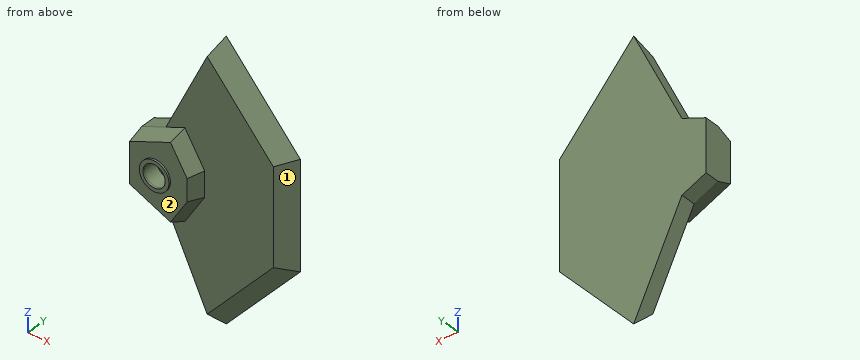
from build123d import *

# Parameters (mm, degrees)
F1_DEPTH      = 8
F1_TAPER      = -20
F2_W          = 14.830423519
F2_H          = 54.1627034545
F3_DEPTH      = 8.0010001
F4_R          = 6
F5_DEPTH      = 8.0010001
F5_DEPTH_BACK = 77
F4_R_2        = 8
F6_DEPTH      = 1
F9_DEPTH      = 8
F10_SIZE      = 7.99999


# Not quite as in the source:
# - a fillet or chamfer is up to 0.001 mm smaller than in the source, because OpenCascade refuses the exact size
# - an extrude ends at something that could not be found from the text; its depth is read off the source's solid


with BuildPart() as f1:
    # F0 (on Front) → F1 (new body)
    with BuildSketch(Plane.XZ):
        Polygon((0, 11), (0, 0), (0, -11), (22.0397368405, -20.5), (31, -6), (31, 0), (31, 6), (22.0397368405, 20.5), align=None)
    extrude(amount=-F1_DEPTH, taper=F1_TAPER)

    # F2 (on Front) → F3 (cut, through all)
    with BuildSketch(Plane.XZ):
        with Locations((-7.4152117595, -1.4976877719)):
            Rectangle(F2_W, F2_H)
    extrude(amount=-F3_DEPTH, mode=Mode.SUBTRACT)

    # F4 (on Front) → F5 (cut, two sides)
    with BuildSketch(Plane.XZ) as f5_sk:
        with Locations((14, 0)):
            Circle(F4_R)
    extrude(amount=-F5_DEPTH, mode=Mode.SUBTRACT)
    extrude(f5_sk.sketch, amount=F5_DEPTH_BACK, mode=Mode.SUBTRACT)

    # F4 (on Front) → F6 (join)
    with BuildSketch(Plane.XZ):
        with Locations((14, 0)):
            Circle(F4_R_2)
        with Locations((14, 0)):
            Circle(F4_R, mode=Mode.SUBTRACT)
    extrude(amount=F6_DEPTH)

    # F8 (on face) → F9 (join)
    with BuildSketch(Plane(origin=(0, 8, 0), x_dir=(-1, 0, 0), z_dir=(0, 1, 0))):
        Polygon((-39, -74.1707404442), (-13, -19.7742556265), (0, -14.1707404442), (0, 14.1707404442), (-13, 19.7742556265), (-39, 74.1707404442), (-78.9322146674, 29), (-78.9322146674, -29), align=None)
    extrude(amount=F9_DEPTH)

    # F10 (size 8 in the source; OpenCascade refuses exactly that, so slightly less here)
    f10_edges = [f1.edges().sort_by_distance(p)[0] for p in [
        (58.966107, 8, 51.58537),
        (78.932215, 8, 0),
        (58.966107, 8, -51.58537),
    ]]
    chamfer(f10_edges, length=F10_SIZE)


solid = f1.part
Can you work these out from the model? Positions are in its coordinate system, mm. Face numbers are marked on the shaded views. A direction names the side the tool comes from. Round coordinates to 2 decimals unless told otherwise and drop trailing zeros. Write each loop counter-clockwise with the first axis right and the second up, starting at its lowest first coordinate (ties: lowest second). Pieces come first, ordered by that corner, then holes. Notation, with made-up numbers: M -2,59 L 52,59 A22 ccw 52,93 Z; hole C 70.25,50.25 d5. An arc over 180 degrees is marked long. Use CSV: the item, a comma, the result in double quotes.
(1) I need wall thicknesses on line 1 along Z through (x, y) = (14, -0.5); line 2 along Y through (x, z) = (56, -22); line 3 along Z through (x, y) = (14, 4). Which ranges of each line are inside material? Lowest first, please.
Check values:
line 1,"-8 to -6, 6 to 8"
line 2,"8 to 16"
line 3,"-18.62 to -6, 6 to 18.62"
(2) I'm going to push flat-ended pins straight in: pin 1 (1.5 mm diameter, centred on y = 3, z = 16, fed in from +X); pin 2 (2 mm diameter, centred on x = 29.5, y = 9, fed in from -Z); pin 3 (3 mm diameter, centred on x = 42, z = -28, fed in from -Y). Where does each tip first touch, or does it pass through?
Check values:
pin 1,"x = 26.67"
pin 2,"z = -56.39"
pin 3,"y = 8"
(3) On a 3-axis mill with a long thin cutter (end or side, diameter ignored), from which of +Z, -Z, +X, -X, +Y, -Y can I reach the whole of each face in a straight line? I mean the marked faces 1 and 2. Say none if no direction works.
Check values:
face 1,"+Z, -Z, +X, -Y"
face 2,"-Y"
(4) Imagine slicing it at A-A (y = 10.25). Write out the boundary of the cut face in (x, z).
Check values:
outline,"M 0,-14.17 L 13,-19.77 L 36.31,-68.54 L 73.18,-26.82 L 73.18,26.82 L 36.31,68.54 L 13,19.77 L 0,14.17 Z"
